Geometry check sheet. Reference: the model listing, model coordinates, mm. Face numbers are marked on the shaded views. Give positions to 0.01 mm unless a question says otherwise; leave off trailing zeros. Order: outer loops, then holes, each group sorted by start corner. A loop starts at its lowest first (then second) coordinate and runs counter-clockwise, first axis right, second up. Notation, with made-up numbers: M -30,56.5 L 14,56.5 A24 ccw 14,88.5 Z; hole C 29,6 d3. An arc over 180 degrees is marked long. Answer as CSV lines item,"result".
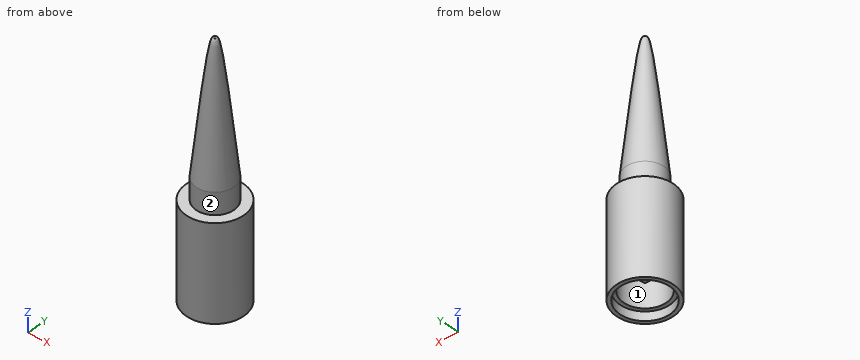
from build123d import *

# Parameters (mm, degrees)
SKETCH1_R           = 9.6
BOSS_EXTRUDE1_DEPTH = 31.71
SKETCH4_R           = 8.42
CUT_EXTRUDE1_DEPTH  = 3.01
SKETCH5_R           = 7.185
CUT_EXTRUDE3_DEPTH  = 12.61
SKETCH6_R           = 2
BOSS_EXTRUDE2_DEPTH = 9.58
CHAMFER1_SIZE       = 1.33
SKETCH7_R           = 6.335
BOSS_EXTRUDE3_DEPTH = 7.22


with BuildPart() as part:
    # Sketch1 → Boss-Extrude1 (new body)
    with BuildSketch(Plane.XY):
        Circle(SKETCH1_R)
    extrude(amount=BOSS_EXTRUDE1_DEPTH)

    # Sketch4 → Cut-Extrude1 (cut)
    with BuildSketch(Plane(origin=(0, 0, 0), x_dir=(-1, 0, 0), z_dir=(0, 0, -1))):
        Circle(SKETCH4_R)
    extrude(amount=-CUT_EXTRUDE1_DEPTH, mode=Mode.SUBTRACT)

    # Sketch5 → Cut-Extrude3 (cut)
    with BuildSketch(Plane(origin=(0, 0, 3.01), x_dir=(-1, 0, 0), z_dir=(0, 0, -1))):
        Circle(SKETCH5_R)
    extrude(amount=-CUT_EXTRUDE3_DEPTH, mode=Mode.SUBTRACT)

    # Sketch6 → Boss-Extrude2 (add)
    with BuildSketch(Plane(origin=(0, 0, 15.62), x_dir=(-1, 0, 0), z_dir=(0, 0, -1))):
        Circle(SKETCH6_R)
    extrude(amount=BOSS_EXTRUDE2_DEPTH)

    # Chamfer1
    chamfer1_edges = [part.edges().sort_by_distance(p)[0] for p in [
        (2, 0, 6.04),
    ]]
    chamfer(chamfer1_edges, length=CHAMFER1_SIZE)

    # Sketch7 → Boss-Extrude3 (add)
    with BuildSketch(Plane.XY.offset(31.71)):
        Circle(SKETCH7_R)
    extrude(amount=BOSS_EXTRUDE3_DEPTH)

    # Sketch10 → Revolve2 (revolve)
    with BuildSketch(Plane(origin=(0, 0, 0), x_dir=(0, 0, -1), z_dir=(1, 0, 0))):
        with BuildLine():
            Line((-81.78, 0), (-38.93, 0))
            Line((-38.93, 0), (-38.93, 6.335))
            add(Edge.make_bspline(
                [(-38.93, 6.335), (-86.441299856, 1.360959474), (-81.78, 0)],
                knots=[0, 0, 0, 1, 1, 1], degree=2, weights=[1, 1.745276846, 1]))
        make_face()
    revolve(axis=Axis((0, 0, 81.78), (0, 0, -1)))


solid = part.part
(1) Draft check along Y on the marked faces 1 and 2. Enter one of: +Y half, -Y half, draft (parallel to the pull), parting line (faces both ways), or undercut.
The answers:
face 1,"undercut"
face 2,"parting line"
(2) Material ranges on line 1 (Y direction, x = 0, z = 12) (3 decimals); line 2 (Y direction, x = 0, z = 1.95); line 3 (X direction, y = 0.75, z = 13), recorded low to high.
The answers:
line 1,"y = -9.6 to -7.185, -2 to 2, 7.185 to 9.6"
line 2,"y = -9.6 to -8.42, 8.42 to 9.6"
line 3,"x = -9.57 to -7.15, -1.85 to 1.85, 7.15 to 9.57"
(3) Section check A-A on z = 14.5. Enter the section's corners in (x, y) (3 decimals), then the cut area to 3 significant figures.
The answers:
outline,"C 0,0 d19.2; C 0,0 d4; hole C 0,0 d14.37"
area,"140 mm2"
(4) Gauge pin test, flat ends, axial feed: P1, Ø1, axis at x = 2.5, z = 41.5, coming from the -Y side; P2, Ø0.7, axis at x = 0, y = 0, coming from the -Z side; P3, Ø5, axis at x = 1.5, y = -4, coming from the -Z side. Record the tip position at first contact, or that the pin passes through.
The answers:
P1,"stops at y = -5.73"
P2,"stops at z = 6.04"
P3,"stops at z = 7.14"
